Work out the finished part from the listing and answer in its coordinate system (mm). Coordinates: 2 decimals unless noted, no trailing zeros. Order: outer loops, then holes, each group sorted by start corner. A loop starts at its lowest first (then second) coordinate and runs counter-clockwise, first axis right, second up. Notation, with made-up numbers: M 18,52.25 L 55,52.25 A25 cw 55,86.25 Z; hole C 74.5,33.25 d2. An arc over 180 degrees is marked long. Write item = value, one per line. Start each with the question number.
Q1. Straight lines are drawn through the part: line 1 along X through (y, z) = (1.95, -62.5); line 2 along X through (y, z) = (1.4, 62.5); line 3 along Z through (x, y) = (40, 1.85). For each, find the intervals that lie inside material, in ascending order.
Q2. Find section B-B on z = -17.5. Give the vertices of the cut face in (x, y).
Q3. Determine the mould class of faces 1 (the flat face through (-1, 0, -1)), 2 (the cylindrical face through (69.533, 1.521, -17.767)) for opening direction Z: released by +Z, released by -Z, zero draft, split by the parting line, or undercut.
Q4. Find section C-C on x = 67.5. Give the vertices of the cut face in (y, z).
Q5. Find section A-A on x = -57.85. Give the vertices of the cut face in (y, z).
Q6. Each of these flat-tipped pins is pushed along its axis until it touches: P1, Ø3.5, axis at x = 22.15, z = -62.5, coming from the +Y side; P2, Ø0.9, axis at x = 62.5, y = 1.5, coming from the -Z side. Where does it stop, or does it pass through?
Q7. Find section D-D on y = 1.8. Give the number of separate pieces and of enclosed holes in the cut face, and give its area (3 significant figures).
```python
from build123d import *

# Parameters (mm, degrees)
SKETCH2_W           = 155
SKETCH2_H           = 145
BOSS_EXTRUDE1_DEPTH = 3
SKETCH4_W           = 40.5
SKETCH4_H           = 10.5
CUT_EXTRUDE1_DEPTH  = 3
SKETCH5_R           = 2.05
CUT_EXTRUDE2_DEPTH  = 3
SKETCH6_R           = 2.05
CUT_EXTRUDE3_DEPTH  = 3


with BuildPart() as part:
    # Sketch2 → Boss-Extrude1 (new body)
    with BuildSketch(Plane(origin=(0, 0, 0), x_dir=(1, 0, 0), z_dir=(0, 1, 0))):
        Rectangle(SKETCH2_W, SKETCH2_H)
    extrude(amount=BOSS_EXTRUDE1_DEPTH)

    # Sketch4 → Cut-Extrude1 (cut)
    with BuildSketch(Plane(origin=(0, 3, 0), x_dir=(1, 0, 0), z_dir=(0, 1, 0))):
        with Locations((57.25, 67.25)):
            Rectangle(SKETCH4_W, SKETCH4_H)
    extrude(amount=-CUT_EXTRUDE1_DEPTH, mode=Mode.SUBTRACT)

    # Sketch5 → Cut-Extrude2 (cut)
    with BuildSketch(Plane(origin=(0, 3, 0), x_dir=(1, 0, 0), z_dir=(0, 1, 0))):
        with Locations(Location((-57.85, 62.5, 0), (0, 0, 270))):
            Circle(SKETCH5_R)
        with Locations(Location((22.15, 62.5, 0), (0, 0, 270))):
            Circle(SKETCH5_R)
        with Locations(Location((47.5, 17.5, 0), (0, 0, 270))):
            Circle(SKETCH5_R)
        with Locations(Location((67.5, 17.5, 0), (0, 0, 270))):
            Circle(SKETCH5_R)
        with Locations(Location((47.5, -62.5, 0), (0, 0, 270))):
            Circle(SKETCH5_R)
        with Locations(Location((67.5, -62.5, 0), (0, 0, 270))):
            Circle(SKETCH5_R)
    extrude(amount=-CUT_EXTRUDE2_DEPTH, mode=Mode.SUBTRACT)

    # Sketch6 → Cut-Extrude3 (cut)
    with BuildSketch(Plane(origin=(0, 3, 0), x_dir=(1, 0, 0), z_dir=(0, 1, 0))):
        with Locations(Location((27.599633374, -52.545679653, 0), (0, 0, 270))):
            Circle(SKETCH6_R)
        with Locations(Location((27.599633374, 41.341825757, 0), (0, 0, 270))):
            Circle(SKETCH6_R)
    extrude(amount=-CUT_EXTRUDE3_DEPTH, mode=Mode.SUBTRACT)


solid = part.part
```
Findings below:
q1.line_1 = -77.5 to -59.9, -55.8 to 20.1, 24.2 to 37
q1.line_2 = -77.5 to 45.45, 49.55 to 65.45, 69.55 to 77.5
q1.line_3 = -62 to 72.5
q2.outline = M -77.5,0 L 45.45,0 L 45.45,3 L -77.5,3 Z; M 49.55,0 L 65.45,0 L 65.45,3 L 49.55,3 Z; M 69.55,0 L 77.5,0 L 77.5,3 L 69.55,3 Z
q3.face_1 = zero draft
q3.face_2 = undercut
q4.outline = M 0,-62 L 3,-62 L 3,-19.55 L 0,-19.55 Z; M 0,-15.45 L 3,-15.45 L 3,60.45 L 0,60.45 Z; M 0,64.55 L 3,64.55 L 3,72.5 L 0,72.5 Z
q5.outline = M 0,-72.5 L 3,-72.5 L 3,-64.55 L 0,-64.55 Z; M 0,-60.45 L 3,-60.45 L 3,72.5 L 0,72.5 Z
q6.P1 = through
q6.P2 = -62
q7.separate_pieces = 1
q7.enclosed_holes = 8
q7.area = 21,900 mm^2
